from build123d import *

# Parameters (mm, degrees)
SKETCH1_W           = 33.655
SKETCH1_H           = 9.525
BOSS_EXTRUDE1_DEPTH = 5.08
SKETCH4_R           = 1.125
CUT_EXTRUDE2_DEPTH  = 20.992418094
FILLET1_R           = 2.54
CUT_EXTRUDE3_DEPTH  = 20.992418094


with BuildPart() as part:
    # Sketch1 → Boss-Extrude1 (new body)
    with BuildSketch(Plane(origin=(0, 0, 0), x_dir=(1, 0, 0), z_dir=(0, 1, 0))):
        Rectangle(SKETCH1_W, SKETCH1_H)
    extrude(amount=BOSS_EXTRUDE1_DEPTH)

    # Sketch4 → Cut-Extrude2 (cut, through all)
    with BuildSketch(Plane.XY.offset(4.7625)):
        with Locations((-14.4325, 2.54)):
            Circle(SKETCH4_R)
    extrude(amount=-CUT_EXTRUDE2_DEPTH, mode=Mode.SUBTRACT)

    # Fillet1
    fillet1_edges = [part.edges().sort_by_distance(p)[0] for p in [
        (-16.8275, 0, 0),
        (-16.8275, 5.08, 0),
    ]]
    fillet(fillet1_edges, radius=FILLET1_R - 0.0001)  # a hair under: the kernel refuses the full size

    # Sketch5 → Cut-Extrude3 (cut, through all)
    with BuildSketch(Plane.XY.offset(4.7625)):
        with BuildLine():
            Line((16.8275, 0), (16.8275, 3.175))
            Line((16.8275, 3.175), (-12.123214396, 3.175))
            ThreePointArc((-12.123214396, 3.175), (-12.05902533, 2.860379446), (-12.0375, 2.54))
            ThreePointArc((-12.0375, 2.54), (-14.4325, 0.145), (-16.8275, 2.54))
            ThreePointArc((-16.8275, 2.54), (-16.083551224, 0.743948776), (-14.2875, 0))
            Line((-14.2875, 0), (16.8275, 0))
        make_face()
    extrude(amount=-CUT_EXTRUDE3_DEPTH, mode=Mode.SUBTRACT)


with BuildPart() as cut_extrude3_kept_piece:
    # of the separate pieces the step leaves, the one the design keeps (cut_extrude3_pieces_kept)
    add(part.part.solids().sort_by_distance((-16.8275, 2.5401, -4.7625))[0])


solid = cut_extrude3_kept_piece.part
Work out the finished part from the listing and answer in its coordinate system (mm). Give positions to 0.01 mm unless a question says otherwise; leave off trailing zeros. Loops run counter-clockwise (first coordinate to the right, second up) from the corner with the lowest first, then second, coordinate; pieces in that order, holes last. Notation, with made-up numbers: M 50.25,17 L 88.25,17 A29 cw 88.25,46 Z; hole C 17.5,67 d3. An arc over 180 degrees is marked long. Use CSV: the item, a comma, the result in double quotes.
1) Find section C-C on x = -8. Write down the section's boundary in (y, z) (1 decimal).
Answer:
outline,"M 3.2,-4.8 L 5.1,-4.8 L 5.1,4.8 L 3.2,4.8 Z"
2) Find section B-B on y = 1.8. Write down the section's boundary in (x, z), plus the area to 4 significant figures.
Answer:
outline,"M -16.71,-4.76 L -15.28,-4.76 L -15.28,4.76 L -16.71,4.76 Z; M -13.59,-4.76 L -12.15,-4.76 L -12.15,4.76 L -13.59,4.76 Z"
area,"27.25 mm^2"
3) Determine the mould class of faces 1 (the cylindrical face through (-15.556, 2.589, 0.067)), 2 (the flat face through (0, 4, -4.762)), 3 (the cylindrical face through (-16.1, 4.32, -0.07)) for opening direction Y: released by +Y, released by -Y, zero draft, split by the parting line, or undercut.
Answer:
face 1,"undercut"
face 2,"zero draft"
face 3,"released by +Y"
4) Given P1, Ø1, axis at y = 4, z = -2.5, coming from the -X side; P2, Ø5, axis at x = 0.5, z = -1, coming from the -Y side (3 decimals), each flat-ended and moving along its own axis, determine where each tip first touches the part or whether it passes through.
Answer:
P1,"x = -16.64"
P2,"y = 3.175"
5) Find section D-D on y = 4.75. Write down the section's boundary in (x, z).
Answer:
outline,"M -15.54,-4.76 L 16.83,-4.76 L 16.83,4.76 L -15.54,4.76 Z"
6) Consider L1, parallel to Y at x = -9.5, z = 3.5 (3 decimals); L2, parallel to X at y = 3.5, z = 2.25; L3, parallel to X at y = 1.7, z = -2.5. Determine where each line is inside the solid, lowest interval first.
Answer:
L1,"3.175 to 5.08"
L2,"-16.64 to -15.02, -13.85 to 16.83"
L3,"-16.68 to -15.18, -13.68 to -12.19"
